Check sheet for the modelled part. Datum: model origin and axes. Units: mm. Give positions to 0.01 mm unless a question says otherwise; leave off trailing zeros. Write each loop counter-clockwise with the first axis right and the second up, starting at its lowest first coordinate (ties: lowest second). Pieces come first, ordered by that corner, then holes. Notation, with made-up numbers: M -25,39.5 L -2,39.5 A25 cw -2,74.5 Z; hole C -27,46.5 d7. An arc over 180 degrees is marked long. Write each question's results on one line, items separated by ' | '. Start each with the question number.
from build123d import *

# Parameters (mm, degrees)
SKETCH1_W           = 10
SKETCH1_H           = 100
BOSS_EXTRUDE1_DEPTH = 10
SKETCH2_R           = 3
SKETCH2_W           = 35
SKETCH2_H           = 70
SKETCH2_H_2         = 35
SKETCH2_H_3         = 90
SKETCH2_H_4         = 134.983592253
SKETCH2_H_5         = 75
CUT_EXTRUDE1_DEPTH  = 10


with BuildPart() as part:
    # Sketch1 → Boss-Extrude1 (new body)
    with BuildSketch(Plane(origin=(0, 0, 0), x_dir=(1, 0, 0), z_dir=(0, 1, 0))):
        Polygon((230, 560), (230, 0), (113, 0), (113, 135), (-200, 135), (-200, 152.241186389), (-230, 152.241186389), (-230, 560), align=None)
        with Locations((120, 265)):
            Rectangle(SKETCH1_W, SKETCH1_H, mode=Mode.SUBTRACT)
        with Locations((-135, 265)):
            Rectangle(SKETCH1_W, SKETCH1_H, mode=Mode.SUBTRACT)
    extrude(amount=BOSS_EXTRUDE1_DEPTH)

    # Sketch2 → Cut-Extrude1 (cut)
    with BuildSketch(Plane.XZ):
        with Locations((215, -470)):
            Circle(SKETCH2_R)
        with Locations((215, -155)):
            Circle(SKETCH2_R)
        with Locations((215, -305)):
            Circle(SKETCH2_R)
        with Locations((-215, -165)):
            Circle(SKETCH2_R)
        with Locations((-215, -470)):
            Circle(SKETCH2_R)
        with Locations((-215, -330)):
            Circle(SKETCH2_R)
        with Locations((81.96618504, -545)):
            Circle(SKETCH2_R)
        with Locations((-86.233971822, -545)):
            Circle(SKETCH2_R)
        with Locations((212.5, -525)):
            Rectangle(SKETCH2_W, SKETCH2_H)
        with Locations((-212.5, -542.5)):
            Rectangle(SKETCH2_W, SKETCH2_H_2)
        with Locations((-212.5, -225)):
            Rectangle(SKETCH2_W, SKETCH2_H_3)
        with Locations((212.5, -67.491796127)):
            Rectangle(SKETCH2_W, SKETCH2_H_4)
        with Locations((212.5, -212.5)):
            Rectangle(SKETCH2_W, SKETCH2_H_5)
        with Locations((212.5, -412.5)):
            Rectangle(SKETCH2_W, SKETCH2_H_5)
    extrude(amount=-CUT_EXTRUDE1_DEPTH, mode=Mode.SUBTRACT)


solid = part.part
Q1. Depth check by flat-ended pin: pin 1 Ø3 at (y, z) = (3, -537.5) entering from -X; pin 2 Ø9.5 at (x, z) = (215, -470) entering from +Y; pin 3 Ø3 at (y, z) = (6.5, -147) entering from -X; pin 4 Ø5 at (x, y) = (214, 6.5) entering from +Z. Enter the tip coordinate at first touch or a pass-through.
Q2. Section check C-C on x = 29.5. Record the boundary of the cut face in (y, z).
Q3. Section check A-A on y = 5.5. State how many separate pieces and enclosed holes the cut face has, plus the area to 3 significant figures.
Q4. Scan lines: L1, parallel to Z at x = -215, y = 7.75; L2, parallel to X at y = 1.75, z = -294.5; L3, parallel to X at y = 3.75, z = -545. Record each from-to range of solid material in increasing order.
Q5. Section check B-B on z = -44. Record the boundary of the cut face in (x, y), plus the area to 3 significant figures.
Check result:
1) pin 1: x = -195 | pin 2: y = 10 | pin 3: x = -200 | pin 4: z = -134.98
2) outline: M 0,-560 L 10,-560 L 10,-135 L 0,-135 Z
3) separate pieces: 1 | enclosed holes: 10 | area: 192,000 mm^2
4) L1: -525 to -473, -467 to -333, -327 to -270, -180 to -168, -162 to -152.24 | L2: -230 to -140, -130 to 115, 125 to 230 | L3: -195 to -89.23, -83.23 to 78.97, 84.97 to 195
5) outline: M 113,0 L 195,0 L 195,10 L 113,10 Z | area: 820 mm^2
